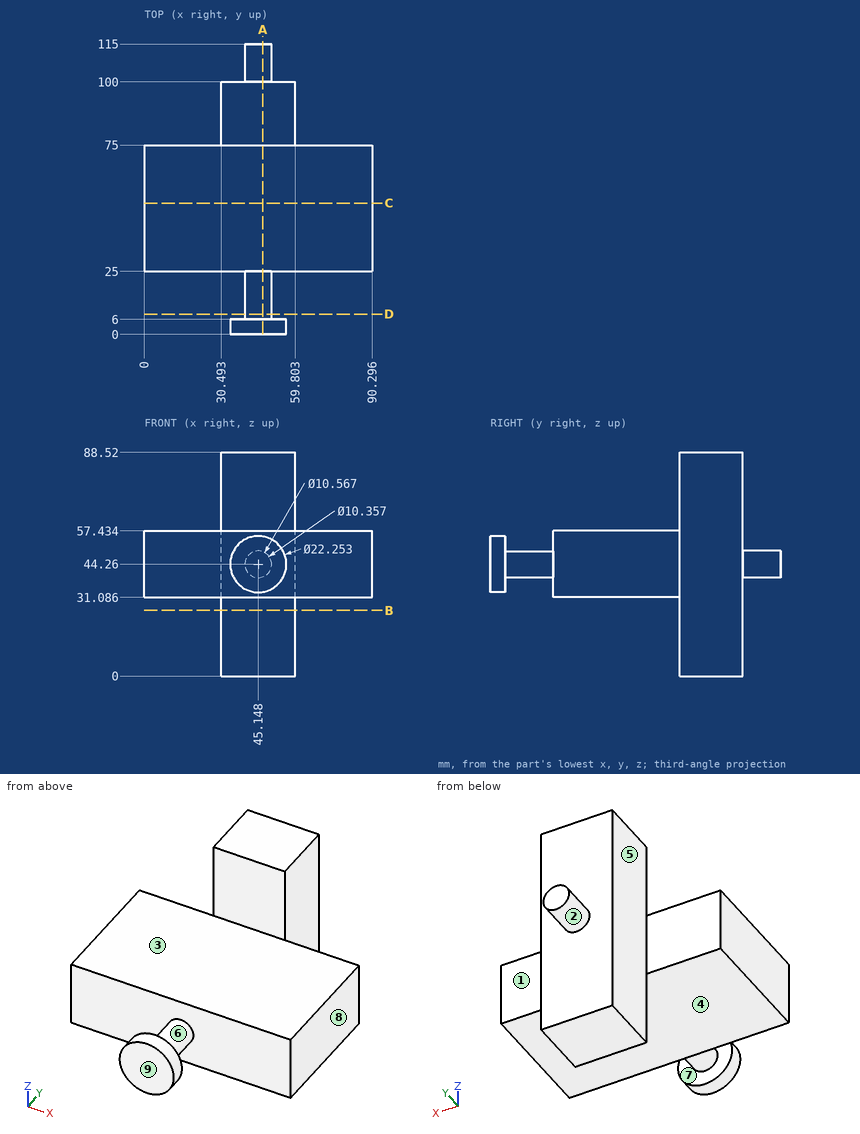
Source: three-view drawing plus pictorial views. Frame: mm from the lowest corner of the part. A direction names the side the tool comes from. Round coordinates to 2 decimals unless told otherwise and drop trailing zeros. Write each loop counter-clockwise with the first axis right and the second up, starting at its lowest first coordinate (ties: lowest second). Pieces come first, ordered by that corner, then holes. Notation, with made-up numbers: M -21.75,-37 L 3.25,-37 A5 ccw 3.25,-28 Z; hole C 21.25,-7.75 d11. An arc over 180 degrees is marked long. Write item = value, one per line.
Item 1: Material intervals for line 1 along Y through (x, z) = (85.5, 54); line 2 along Z through (x, y) = (33.5, 68.5) (1 decimal); line 3 along Y through (x, z) = (53, 51), sorted ascending. Write a range as [from, to].
Findings:
line_1 = [25, 75]
line_2 = [31.1, 57.4]
line_3 = [0, 6], [25, 100]
Item 2: Pull-direction query (Y, two-part tool) for the marked faces 6, 7, 8 and 9; classes: pulls with the +Y half, pulls with the -Y half, needs draft (parallel to the pull), parting line crosses it, or undercut.
Findings:
face_6 = undercut
face_7 = undercut
face_8 = needs draft
face_9 = pulls with the -Y half
Item 3: Access query for the marked faces 1, 2, 3, 4 and 5. Directions: +Z, -Z, +X, -X, +Y, -Y. A direction counts if a zero-diameter tool reaches every point of the face in a straight line with its end or side. Return the directions, or none.
Findings:
face_1 = +Z, -Z, +X, +Y
face_2 = +Y
face_3 = +Z, +X, -X, -Y
face_4 = -Z, +X, -X, -Y
face_5 = +Z, -Z, -X, +Y
Item 4: Section query C-C on y = 52. Return loops of the section in (x, z) (1 decimal).
Findings:
outline = M 0,31.1 L 90.3,31.1 L 90.3,57.4 L 0,57.4 Z
Item 5: Pin query (flat end, axial travel): P1, Ø3, axis at x = 52.5, y = 57.5, coming from the +Z side; P2, Ø15, axis at x = 23.5, y = 42, coming from the -Z side; P3, Ø13, axis at x = 14.5, z = 46.5, coming from the +Y side; P4, Ø11, axis at x = 50.5, z = 49.5, coming from the +Y side. Return the tip coordinate at first contact, or that it passes through.
Findings:
P1 = 57.43
P2 = 31.09
P3 = 75
P4 = 115
Item 6: Section query A-A on x = 47. Return loops of the section in (y, z) (1 decimal).
Findings:
outline = M 0,33.3 L 6,33.3 L 6,39.4 L 25,39.4 L 25,31.1 L 75,31.1 L 75,0 L 100,0 L 100,39.3 L 115,39.3 L 115,49.2 L 100,49.2 L 100,88.5 L 75,88.5 L 75,57.4 L 25,57.4 L 25,49.1 L 6,49.1 L 6,55.2 L 0,55.2 Z
Item 7: Section query D-D on y = 8. Return loops of the section in (x, z).
Findings:
outline = C 45.15,44.26 d10.36
Item 8: Section query B-B on z = 26. Return loops of the section in (x, y).
Findings:
outline = M 30.49,75 L 59.8,75 L 59.8,100 L 30.49,100 Z
